from build123d import *

# Parameters (mm, degrees)
SKETCH1_W           = 50.8
SKETCH1_H           = 50.8
BOSS_EXTRUDE1_DEPTH = 38.1
SKETCH2_R           = 16.383
CUT_EXTRUDE1_DEPTH  = 49.53
CUT_EXTRUDE2_DEPTH  = 29.21


with BuildPart() as part:
    # Sketch1 → Boss-Extrude1 (new body)
    with BuildSketch(Plane(origin=(0, 0, 0), x_dir=(1, 0, 0), z_dir=(0, 1, 0))):
        Rectangle(SKETCH1_W, SKETCH1_H)
    extrude(amount=BOSS_EXTRUDE1_DEPTH)

    # Sketch2 → Cut-Extrude1 (cut)
    with BuildSketch(Plane(origin=(0, 38.1, 0), x_dir=(1, 0, 0), z_dir=(0, 1, 0))):
        with Locations(Location((0, 0, 0), (0, 0, 270))):
            Circle(SKETCH2_R)
    extrude(amount=-CUT_EXTRUDE1_DEPTH, mode=Mode.SUBTRACT)

    # Sketch3 → Cut-Extrude2 (cut)
    with BuildSketch(Plane(origin=(25.4, 0, 0), x_dir=(0, 0, -1), z_dir=(1, 0, 0))):
        with BuildLine():
            Line((-7.718095527, 9.445615075), (7.718095527, 9.445615075))
            ThreePointArc((7.718095527, 9.445615075), (9.514146751, 8.701666299), (10.258095527, 6.905615075))
            Line((10.258095527, 6.905615075), (10.258095527, 5.424599661))
            ThreePointArc((10.258095527, 5.424599661), (9.514146751, 3.628548437), (7.718095527, 2.884599661))
            Line((7.718095527, 2.884599661), (-7.718095527, 2.884599661))
            ThreePointArc((-7.718095527, 2.884599661), (-9.514146751, 3.628548437), (-10.258095527, 5.424599661))
            Line((-10.258095527, 5.424599661), (-10.258095527, 6.905615075))
            ThreePointArc((-10.258095527, 6.905615075), (-9.514146751, 8.701666299), (-7.718095527, 9.445615075))
        make_face()
    extrude(amount=-CUT_EXTRUDE2_DEPTH, mode=Mode.SUBTRACT)


solid = part.part
Read the model definition and answer for the solid it produces. Units are mm, in the model's axes. A direction names the side the tool comes from. Give positions to 0.01 mm unless a question says otherwise; leave off trailing zeros. Loops run counter-clockwise (first coordinate to the right, second up) from the corner with the lowest first, then second, coordinate; pieces in that order, holes last. Notation, with made-up numbers: (-27.5, 4.25) -> (-16.5, 4.25) arc R17 cw to (-16.5, 36.25) -> close; hole circle Ø2 at (-12, 58). An arc over 180 degrees is marked (long way). Answer as CSV lines item,"result".
Item 1: This flat-tipped pin is pushed along its axis until it touches: pin 1 (8 mm diameter, centred on x = -1, z = 10.5, fed in from +Y). Where does it stop, or does it pass through?
Returned:
pin 1,"passes through"
Item 2: For faces 4 (the face through (19.175, 8.682, 9.534)), 5 (the face through (0, 19, -25.4)), determine the directions among +Z, -Z, +X, -X, +Y, -Y from which every point of the face is accessible in a straight line to the end or side of a thin tool.
Returned:
face 4,"+X"
face 5,"-Z, +X, -X, +Y, -Y"
Item 3: Find section B-B on z = 0. Give the vertices of the cut face in (x, y).
Returned:
outline,"(-25.4, 0) -> (-16.38, 0) -> (-16.38, 38.1) -> (-25.4, 38.1) -> close; (16.38, 0) -> (25.4, 0) -> (25.4, 2.88) -> (16.38, 2.88) -> close; (16.38, 9.45) -> (25.4, 9.45) -> (25.4, 38.1) -> (16.38, 38.1) -> close"
Item 4: Determine the mould class of faces 1 (the face through (19.175, 3.609, 9.494)), 2 (the face through (25.4, 19, 0)), 3 (the face through (-12, 38.1, -12)) for opening direction Y: +Y half, -Y half, draft (parallel to the pull), parting line (faces both ways), or undercut.
Returned:
face 1,"undercut"
face 2,"draft"
face 3,"+Y half"
Item 5: Find section C-C on y = 27.5. Give the vertices of the cut face in (x, z).
Returned:
outline,"(-25.4, -25.4) -> (25.4, -25.4) -> (25.4, 25.4) -> (-25.4, 25.4) -> close; hole circle Ø32.77 at (0, 0)"
Item 6: Find section A-A on x = 0. Give the vertices of the cut face in (y, z).
Returned:
outline,"(0, -25.4) -> (38.1, -25.4) -> (38.1, -16.38) -> (0, -16.38) -> close; (0, 16.38) -> (38.1, 16.38) -> (38.1, 25.4) -> (0, 25.4) -> close"
Item 7: Consider line 1 (X direction, y = 17, z = 0); line 2 (X direction, y = 34, z = -11.5); line 3 (Z direction, x = 6.5, y = 8.5). Determine where each line is inside the solid, lowest interval first. Write a range as [from, to].
Returned:
line 1,"x = [-25.4, -16.38], [16.38, 25.4]"
line 2,"x = [-25.4, -11.67], [11.67, 25.4]"
line 3,"z = [-25.4, -15.04], [15.04, 25.4]"
Item 8: Find section D-D on z = -9.5. Give the vertices of the cut face in (x, y), plus the area to 3 significant figures.
Returned:
outline,"(-25.4, 0) -> (-13.35, 0) -> (-13.35, 38.1) -> (-25.4, 38.1) -> close; (13.35, 0) -> (25.4, 0) -> (25.4, 3.61) -> (13.35, 3.61) -> close; (13.35, 8.72) -> (25.4, 8.72) -> (25.4, 38.1) -> (13.35, 38.1) -> close"
area,"857 mm²"
